from build123d import *

# Parameters (mm, degrees)
BASPROSKE_W     = 30
BASPROSKE_H     = 80
TOOTHCUT_DEPTH  = 118.046999107
TEETHCUTS_COUNT = 30
TEETHCUTS_ANGLE = 348
BORSKE_W        = 30
BORSKE_H        = 30
BORE_DEPTH      = 50.0000508


with BuildPart() as part:
    # BasProSke → Base-Revolve (revolve)
    with BuildSketch(Plane(origin=(0, 0, 0), x_dir=(1, 0, 0), z_dir=(0, 1, 0)), mode=Mode.PRIVATE) as base_revolve_sk:
        with Locations((15, 40)):
            Rectangle(BASPROSKE_W, BASPROSKE_H)
    revolve(base_revolve_sk.sketch.rotate(Axis((-10, 0, 0), (1, 0, 0)), 180), axis=Axis((-10, 0, 0), (1, 0, 0)))

    # TooCutSke → ToothCut (cut, through all)
    with BuildSketch(Plane(origin=(0, 0, 0), x_dir=(0, 0, -1), z_dir=(1, 0, 0))):
        with BuildLine():
            ThreePointArc((2.295869197, 68.710654091), (0, 68.749), (-2.295869197, 68.710654091))
            ThreePointArc((-2.295869197, 68.710654091), (-4.034057509, 74.450113805), (-6.879070213, 79.729185611))
            ThreePointArc((-6.879070213, 79.729185611), (0, 80.0254), (6.879070213, 79.729185611))
            ThreePointArc((6.879070213, 79.729185611), (4.034057509, 74.450113805), (2.295869197, 68.710654091))
        make_face()
    toothcut = extrude(amount=TOOTHCUT_DEPTH, mode=Mode.SUBTRACT)

    # TeethCuts: ToothCut ×30 about axis
    teethcuts_axis = Axis((-10, 0, 0), (1, 0, 0))
    for i in range(1, TEETHCUTS_COUNT):
        add(toothcut.rotate(teethcuts_axis, i * TEETHCUTS_ANGLE / (TEETHCUTS_COUNT - 1)), mode=Mode.SUBTRACT)

    # BorSke → Bore (cut, symmetric)
    with BuildSketch(Plane(origin=(0, 0, 0), x_dir=(0, 0, -1), z_dir=(1, 0, 0))):
        Rectangle(BORSKE_W, BORSKE_H)
    extrude(amount=BORE_DEPTH, both=True, mode=Mode.SUBTRACT)


solid = part.part
Could you check a few things on this model? Use its own coordinates, in mm. A direction names the side the tool comes from. Give positions to 0.01 mm unless a question says otherwise; leave off trailing zeros. Order: outer loops, then holes, each group sorted by start corner. A loop starts at its lowest first (then second) coordinate and runs counter-clockwise, first axis right, second up. Notation, with made-up numbers: (68.25, 25.25) - (112.25, 25.25) arc R12 cw to (112.25, 45.25) - close; hole circle Ø3 at (53.25, 48). An arc over 180 degrees is marked (long way). Return JSON: item names as keys, results as strings. Group by question number.
Q1. Thinking about a two-plate mould opening in Z: for faces 1 (the face through (14.79, -55.64, -40.38)), 2 (the face through (0, -1, -17)), 3 (the face through (14.79, -26.888, -69.612)), 4 (the face through (14.79, -67.24, 14.33)), which applies, pulls with the +Z half, pulls with the -Z half, needs draft (parallel to the pull), parting line crosses it, or undercut?
Q2. Suppose I cut it at C-C, the plane y = 13. Please give me the cut outline in (x, z).
Q3. Suppose I cut it at D-D, the plane z = -33.5. Please give me the cut outline in (x, y).
Q4. Please list where these lines run through material, in increasing order: line 1 along Y through (x, z) = (15.5, 59); line 2 along Y through (x, z) = (26.75, -51); line 3 along Z through (x, y) = (20, -59.5). Write a range as [from, to].
Q5. Which directions (+Z, -Z, +X, -X, +Y, -Y) give clear straight access to the entire face, cutting with the end or side of a thin tool? Please do faces 5 (the face through (14.79, 57.81, 46.94)), 6 (the face through (14.79, -26.779, 69.485)), 7 (the face through (14.79, 46.786, 57.934)).
Q6. Will these pins go through, and if not, where does the flat tip stop? pin 1 Ø1.5 at (x, z) = (26.5, 52) entering from +Y; pin 2 Ø1.5 at (x, y) = (18, -17) entering from +Z; pin 3 Ø2 at (x, y) = (6.5, -30) entering from +Z.
Q7. Suppose I cut it at A-A, the plane y = -7.5. Please give me the cut outline in (x, z), and give its area (3 significant figures).
Q8. Suppose I cut it at B-B, the plane z = 46.5. Please give me the cut outline in (x, y), and give its area (3 significant figures).
Resolved:
{
 "1": {"face 1": "undercut", "face 2": "needs draft", "face 3": "pulls with the -Z half", "face 4": "undercut"},
 "2": {"outline": "(0, -75.64) - (30, -75.64) - (30, -15) - (0, -15) - close; (0, 15) - (30, 15) - (30, 75.64) - (0, 75.64) - close"},
 "3": {"outline": "(0, -65.92) - (30, -65.92) - (30, 65.92) - (0, 65.92) - close"},
 "4": {"line 1": "y = [-47.14, -36.92], [-35.29, 35.29], [36.92, 47.14]", "line 2": "y = [-59.9, -49.84], [-46.1, 46.1], [49.84, 59.9]", "line 3": "z = [-53.48, -50.1], [-39.58, 39.58], [50.1, 53.48]"},
 "5": {"face 5": "+X, -X, +Y", "face 6": "+Z, +X, -X", "face 7": "+X, -X"},
 "6": {"pin 1": "stops at y = 60.45", "pin 2": "stops at z = 78.33", "pin 3": "stops at z = 73.56"},
 "7": {"outline": "(0, -68.34) - (30, -68.34) - (30, -15) - (0, -15) - close; (0, 15) - (30, 15) - (30, 68.34) - (0, 68.34) - close", "area": "3,200 mm2"},
 "8": {"outline": "(0, -57.53) - (30, -57.53) - (30, 57.53) - (0, 57.53) - close", "area": "3,450 mm2"}
}
